Build history of the part. All positions in model axes, mm. A direction names the side the tool comes from. Round coordinates to 2 decimals unless told otherwise and drop trailing zeros. Loops run counter-clockwise (first coordinate to the right, second up) from the corner with the lowest first, then second, coordinate; pieces in that order, holes last. Notation, with made-up numbers: (8, -9) - (46, -9) arc R18 ccw to (46, 19) - close; hole circle Ø7 at (-40, -35.75). An arc over 180 degrees is marked (long way). One line per question, with ' | ' between items. Start each with the question number.
from build123d import *

# Parameters (mm, degrees)
EXTRUDE_1_DEPTH     = 3
CUT_EXTRUDE_1_DEPTH = 39.366652187


with BuildPart() as part:
    # 草图1 → 凸台-拉伸1 (new body)
    with BuildSketch(Plane.XY):
        Polygon((16, 0), (8, 13.856406461), (-8, 13.856406461), (-16, 0), (-8, -13.856406461), (8, -13.856406461), align=None)
    extrude(amount=EXTRUDE_1_DEPTH)

    # 草图2 → 旋转1 (revolve)
    with BuildSketch(Plane(origin=(0, 0, 0), x_dir=(0, 0, -1), z_dir=(1, 0, 0)), mode=Mode.PRIVATE) as revolve_1_sk:
        Polygon((0, 0), (0, 7), (2, 7), (2, 9), (30, 9), (32, 7), (32, 0), align=None)
    revolve(revolve_1_sk.sketch.rotate(Axis((0, 0, -32), (0, 0, 1)), 90), axis=Axis((0, 0, -32), (0, 0, 1)))

    # 草图4 → 切除-拉伸1 (cut, through all)
    with BuildSketch(Plane.XY):
        Polygon((16, 0), (8, 13.856406461), (-8, 13.856406461), (-16, 0), (-8, -13.856406461), (8, -13.856406461), align=None)
        Polygon((12, 0), (6, 10.392304845), (-6, 10.392304845), (-12, 0), (-6, -10.392304845), (6, -10.392304845), align=None, mode=Mode.SUBTRACT)
    extrude(amount=CUT_EXTRUDE_1_DEPTH, mode=Mode.SUBTRACT)


solid = part.part
1) Drop flat-ended pins along their axis: pin 1 (5 mm diameter, centred on y = 7, z = -7.5, fed in from -X); pin 2 (10 mm diameter, centred on y = 0.5, z = -20, fed in from +X); pin 3 (1.5 mm diameter, centred on y = -2.5, z = -21.5, fed in from +X). Give the stop position or say it passes through.
2) Two-plate mould, pull along Z, no slides. Class faces 1 (the flat face through (0, 7.3, -2)), 2 (the flat face through (0, 0, 3)), 3 (the flat face through (0, 0, -32)): +Z half, -Z half, draft (parallel to the pull), parting line (faces both ways), or undercut.
3) Wall check: line 1 (Z direction, x = 5.5, y = -7); line 2 (X direction, y = 0.25, z = -11.5); line 3 (Y direction, x = 5.25, z = -10.5). Give the ranges that are in metal, low to high. Write a range as [from, to].
4) Saw through at B-B on z = -18. Write the cut outline in (x, y), and give its area (3 significant figures).
5) Saw through at A-A on x = 0. Write the cut outline in (y, z), and give its area (3 significant figures).
6) Tool access for faces 4 (the cylindrical face through (6.633, -6.083, -16.196)), 5 (the flat face through (-8.958, 5.269, 1.479)), 6 (the cylindrical face through (-3.23, 6.21, -1.01)): list every direction of +Z, -Z, +X, -X, +Y, -Y with a clear straight run to the whole face (end or side of a thin tool).
Answer key:
1) pin 1: x = -7.79 | pin 2: x = 9 | pin 3: x = 8.83
2) face 1: undercut | face 2: +Z half | face 3: -Z half
3) line 1: [-30.1, -2], [0, 3] | line 2: [-9, 9] | line 3: [-7.31, 7.31]
4) outline: circle Ø18 at (0, 0) | area: 254 mm²
5) outline: (-10.39, 0) - (-7, 0) - (-7, -2) - (-9, -2) - (-9, -30) - (-7, -32) - (7, -32) - (9, -30) - (9, -2) - (7, -2) - (7, 0) - (10.39, 0) - (10.39, 3) - (-10.39, 3) - close | area: 626 mm²
6) face 4: -Z | face 5: +Z, -Z, -X, +Y | face 6: none
